Verification items for the finished model (mm, model axes). A direction names the side the tool comes from. Round coordinates to 2 decimals unless told otherwise and drop trailing zeros. Write each loop counter-clockwise with the first axis right and the second up, starting at its lowest first coordinate (ties: lowest second). Pieces come first, ordered by that corner, then holes.
from build123d import *

# Parameters (mm, degrees)
EXTRUDE_1_DEPTH     = 30
SKETCH_2_R          = 3
CUT_EXTRUDE_1_DEPTH = 60
SKETCH_3_R          = 5
CUT_EXTRUDE_2_DEPTH = 60


with BuildPart() as part:
    # 스케치1 → 보스-돌출1 (new body)
    with BuildSketch(Plane.XY):
        Polygon((0, 0), (0, 60), (60, 0), align=None)
    extrude(amount=EXTRUDE_1_DEPTH)

    # 스케치2 → 컷-돌출1 (cut)
    with BuildSketch(Plane.ZY):
        with Locations((15, 15)):
            Circle(SKETCH_2_R)
        with Locations((15, 45)):
            Circle(SKETCH_2_R)
    extrude(amount=-CUT_EXTRUDE_1_DEPTH, mode=Mode.SUBTRACT)

    # 스케치3 → 컷-돌출2 (cut)
    with BuildSketch(Plane.ZY.offset(-5)):
        with Locations((15, 15)):
            Circle(SKETCH_3_R)
        with Locations((15, 45)):
            Circle(SKETCH_3_R)
    extrude(amount=-CUT_EXTRUDE_2_DEPTH, mode=Mode.SUBTRACT)


solid = part.part
Q1. Tool access check on faces 5 (the cylindrical face through (10.73, 40.12, 13.92)), 6 (the flat face through (0, 30, 15)). Record the directions out of +Z, -Z, +X, -X, +Y, -Y that give a thin tool (end or side, any length) a straight path to the whole face; none if there is none.
Recorded:
face 5: +X
face 6: +Z, -Z, -X, +Y, -Y
Q2. Sectioned sample at D-D (x = 48). Enter the section's corners in (y, z), plus the area to 3 significant figures.
Recorded:
outline: (0, 0) - (12, 0) - (12, 11) arc R5 cw to (12, 19) - (12, 30) - (0, 30) - close
area: 349 mm2
Q3. Sectioned sample at A-A (z = 15). Enter the section's corners in (x, y), plus the area to 3 significant figures.
Recorded:
outline: (0, 0) - (60, 0) - (50, 10) - (5, 10) - (5, 12) - (0, 12) - close; (0, 18) - (5, 18) - (5, 20) - (40, 20) - (20, 40) - (5, 40) - (5, 42) - (0, 42) - close; (0, 48) - (5, 48) - (5, 50) - (10, 50) - (0, 60) - close
area: 1,240 mm2
Q4. Sectioned sample at C-C (y = 43.5). Enter the section's corners in (x, z), plus the area to 3 significant figures.
Recorded:
outline: (0, 0) - (16.5, 0) - (16.5, 10.23) - (5, 10.23) - (5, 12.4) - (0, 12.4) - close; (0, 17.6) - (5, 17.6) - (5, 19.77) - (16.5, 19.77) - (16.5, 30) - (0, 30) - close
area: 359 mm2
Q5. Sectioned sample at B-B (x = 40). Enter the section's corners in (y, z), plus the area to 3 significant figures.
Recorded:
outline: (0, 0) - (20, 0) - (20, 30) - (0, 30) - close; hole circle Ø10 at (15, 15)
area: 521 mm2
Q6. Depth check by flat-ended pin: P1, Ø4, axis at y = 40, z = 14, coming from the +X side; P2, Ø8, axis at y = 46, z = 13, coming from the +X side; P3, Ø3, axis at y = 20, z = 10.5, coming from the +X side; P4, Ø3, axis at x = 14.5, z = 9.5, coming from the -Y side. Enter the tip coordinate at first touch or a pass-through.
Recorded:
P1: stops at x = 22
P2: stops at x = 17.09
P3: stops at x = 41.5
P4: stops at y = 0
Q7. Release check for a two-part mould opening along Y. For faces 1 (the flat face through (17, 17, 0)), 2 (the cylindrical face through (27.18, 10.12, 13.92)), 3 (the flat face through (30, 30, 15)), 4 (the cylindrical face through (2, 48, 15)) record: released by +Y, released by -Y, zero draft, split by the parting line, or undercut.
Recorded:
face 1: zero draft
face 2: undercut
face 3: released by +Y
face 4: undercut
Q8. Material ranges on line 1 along Y through (x, z) = (3, 15); line 2 along Y through (x, z) = (3.7, 15); line 3 along X through (y, z) = (18, 10), recorded low to high.
Recorded:
line 1: y = 0 to 12, 18 to 42, 48 to 57
line 2: y = 0 to 12, 18 to 42, 48 to 56.3
line 3: x = 0 to 42
